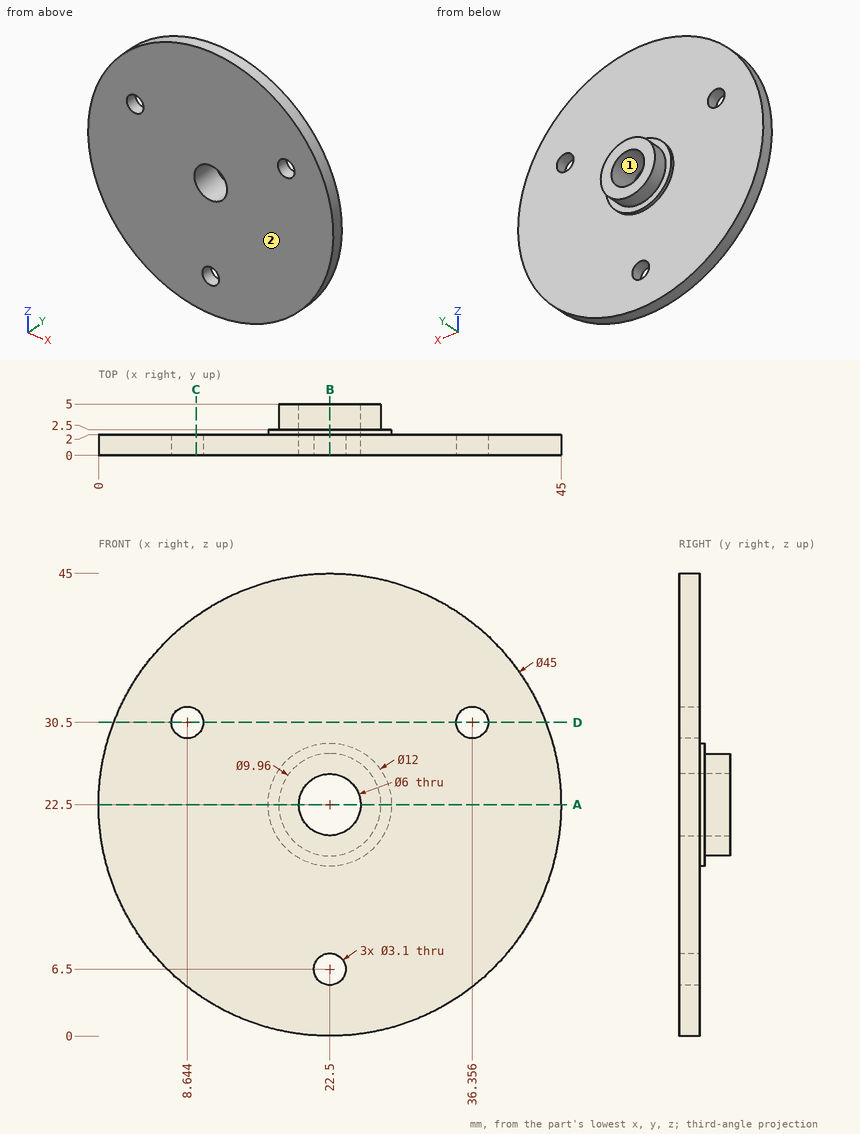
Design review of the part shown in the three views and the two pictorial views. Dimensions are in mm from the part's minimum x, y and z. Give positions to 0.01 mm unless a question says otherwise; leave off trailing zeros. Write each loop counter-clockwise with the first axis right and the second up, starting at its lowest first coordinate (ties: lowest second). Pieces come first, ordered by that corner, then holes. Notation, with made-up numbers: M 33.25,-2 L 89.25,-2 A31 ccw 89.25,26 Z; hole C 52,45.5 d6. An arc over 180 degrees is marked long. Answer in a Markdown table with one row per item.
Item 1: Add section B-B on x = 22.5. Give the boundary of the cut face in (y, z).
Check sheet entries:
| item | result |
|---|---|
| outline | M 0,0 L 2,0 L 2,4.95 L 0,4.95 Z; M 0,8.05 L 2,8.05 L 2,16.5 L 2.5,16.5 L 2.5,17.52 L 5,17.52 L 5,19.5 L 0,19.5 Z; M 0,25.5 L 5,25.5 L 5,27.48 L 2.5,27.48 L 2.5,28.5 L 2,28.5 L 2,45 L 0,45 Z |
Item 2: Add section C-C on x = 9.5. Give the boundary of the cut face in (y, z) (1 decimal).
Check sheet entries:
| item | result |
|---|---|
| outline | M 0,4.1 L 2,4.1 L 2,29.2 L 0,29.2 Z; M 0,31.8 L 2,31.8 L 2,40.9 L 0,40.9 Z |
Item 3: Add section A-A on z = 22.5. Give the boundary of the cut face in (x, y).
Check sheet entries:
| item | result |
|---|---|
| outline | M 0,0 L 19.5,0 L 19.5,5 L 17.52,5 L 17.52,2.5 L 16.5,2.5 L 16.5,2 L 0,2 Z; M 25.5,0 L 45,0 L 45,2 L 28.5,2 L 28.5,2.5 L 27.48,2.5 L 27.48,5 L 25.5,5 Z |
Item 4: For P1, Ø13.5, axis at x = 13, z = 32, coming from the +Y side; P2, Ø1, axis at x = 25, y = 3.5, coming from the +Z side; P3, Ø9.5, axis at x = 23.5, z = 20, coming from the +Y side; P4, Ø3.5, axis at x = 22.5, z = 22.5, coming from the -Y side, all flat-tipped, find the tip position at first contact; note any pin that passes through.
Check sheet entries:
| item | result |
|---|---|
| P1 | y = 2 |
| P2 | z = 27.06 |
| P3 | y = 5 |
| P4 | through |
Item 5: Draft analysis for pull direction Z (two halves, no side actions). For the marked faces 1 and 2, state which applies: +Z half, -Z half, draft (parallel to the pull), parting line (faces both ways), or undercut.
Check sheet entries:
| item | result |
|---|---|
| face 1 | undercut |
| face 2 | draft |
Item 6: Add section D-D on z = 30.5. Give the boundary of the cut face in (x, y).
Check sheet entries:
| item | result |
|---|---|
| outline | M 1.47,0 L 7.09,0 L 7.09,2 L 1.47,2 Z; M 10.19,0 L 34.81,0 L 34.81,2 L 10.19,2 Z; M 37.91,0 L 43.53,0 L 43.53,2 L 37.91,2 Z |
Item 7: For line 1 along X through (y, z) = (1.1, 30.5) (1 decimal); line 2 along Y through (x, z) = (13.5, 33); line 3 along Z through (x, y) = (21, 2.25), list the stretches that pass through material, from the lowest coordinate up.
Check sheet entries:
| item | result |
|---|---|
| line 1 | 1.5 to 7.1, 10.2 to 34.8, 37.9 to 43.5 |
| line 2 | 0 to 2 |
| line 3 | 16.69 to 19.9, 25.1 to 28.31 |
